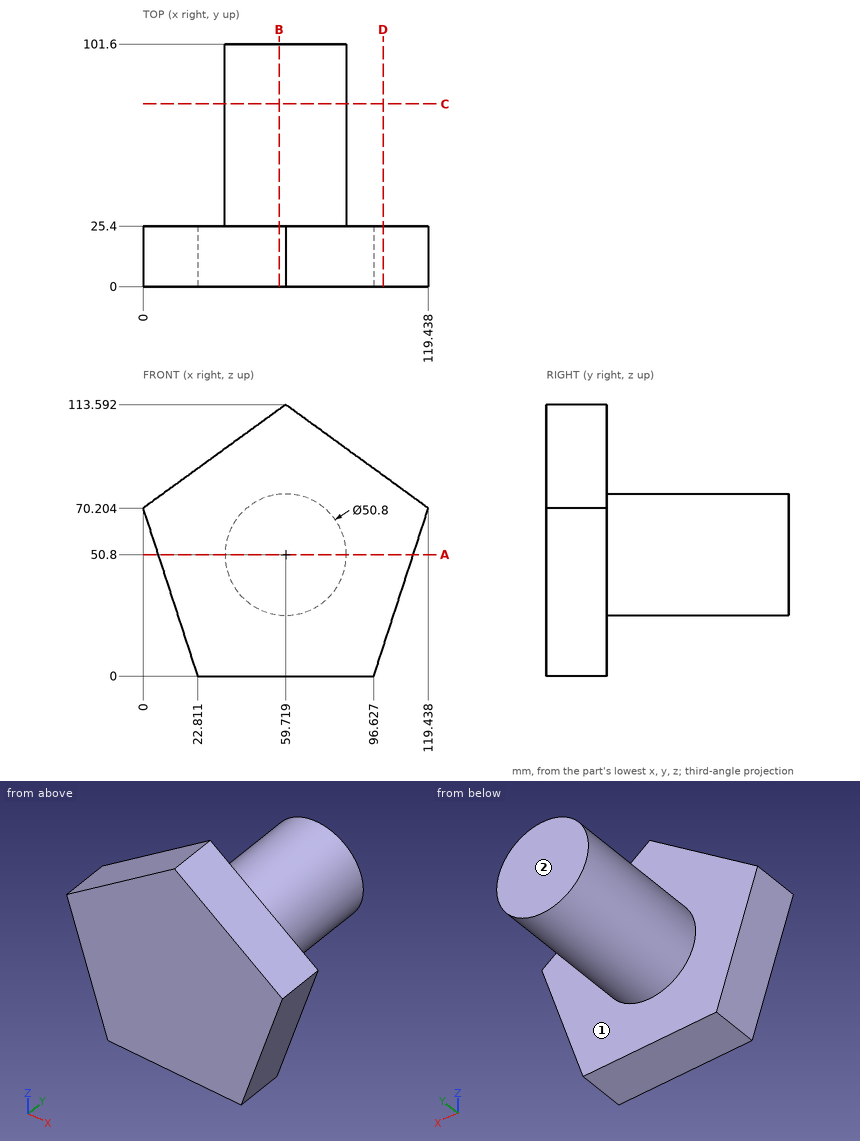
Part print with two shaded views. Sizes in mm from the minimum x, y, z corner. A direction names the side the tool comes from. Round coordinates to 2 decimals unless told otherwise and drop trailing zeros. Order: outer loops, then holes, each group sorted by start corner. A loop starts at its lowest first (then second) coordinate and runs counter-clockwise, first axis right, second up. Notation, with made-up numbers: M 48,56.25 L 80,56.25 A21 ccw 80,76.25 Z; hole C 72.5,-5 d5. An arc over 180 degrees is marked long. Answer in a Markdown table with one row per item. Add a question column.
Q1. Cut at B-B on x = 57. Give the cut face in (y, z).
Q2. Cut at C-C on y = 76.5. Give the cut face in (x, z).
Q3. 3-axis set-ups, long thin cutter, end or side, ignore diameter. For the marked faces 1 and 2: which of +Z, -Z, +X, -X, +Y, -Y reach the whole face in a straight line?
Q4. Pin check, flat tips, straight feed: pin 1 (8 mm diameter, centred on x = 84.5, y = 35.5, fed in from +Z) (1 decimal); pin 2 (5 mm diameter, centred on x = 28.5, y = 19, fed in from -Z); pin 3 (6 mm diameter, centred on x = 54.5, y = 86.5, fed in from -Z); pin 4 (3 mm diameter, centred on x = 61, y = 52.5, fed in from +Z). Stop position of each tip, or through.
Q5. Cut at D-D on x = 100.5. Give the cut face in (y, z), and give its area (3 significant figures).
Q6. Wall check: L1, parallel to Y at x = 81, z = 85.5; L2, parallel to Z at x = 59.5, y = 43; L3, parallel to X at y = 19.5, z = 96 (1 decimal). Give the ranges that are in metal, low to high. Write a range as from..to.
Q7. Cut at A-A on z = 50.8. Give the cut face in (x, y) (1 decimal), and give its area (3 significant figures).
Established:
| question | item | result |
|---|---|---|
| 1 | outline | M 0,0 L 25.4,0 L 25.4,25.55 L 101.6,25.55 L 101.6,76.05 L 25.4,76.05 L 25.4,111.62 L 0,111.62 Z |
| 2 | outline | C 59.72,50.8 d50.8 |
| 3 | face 1 | +Y |
| 3 | face 2 | +Z, -Z, +X, -X, +Y |
| 4 | pin 1 | stops at z = 65.4 |
| 4 | pin 2 | stops at z = 0 |
| 4 | pin 3 | stops at z = 25.5 |
| 4 | pin 4 | stops at z = 76.2 |
| 5 | outline | M 0,11.92 L 25.4,11.92 L 25.4,83.96 L 0,83.96 Z |
| 5 | area | 1,830 mm2 |
| 6 | L1 | y = 0..25.4 |
| 6 | L2 | z = 25.4..76.2 |
| 6 | L3 | x = 35.5..83.9 |
| 7 | outline | M 6.3,0 L 113.1,0 L 113.1,25.4 L 85.1,25.4 L 85.1,101.6 L 34.3,101.6 L 34.3,25.4 L 6.3,25.4 Z |
| 7 | area | 6,580 mm2 |
